For this review, use the dimensioned drawing (mm, ordinates from the lowest corner) and the shaded views. A direction names the side the tool comes from. Coordinates: 2 decimals unless noted, no trailing zeros. Loops run counter-clockwise (first coordinate to the right, second up) from the corner with the lowest first, then second, coordinate; pieces in that order, holes last. Notation, with made-up numbers: M 7,30.5 L 39,30.5 A30 ccw 39,66.5 Z; hole C 76.5,32.25 d8. An arc over 180 degrees is marked long. One line per item, written item: value.
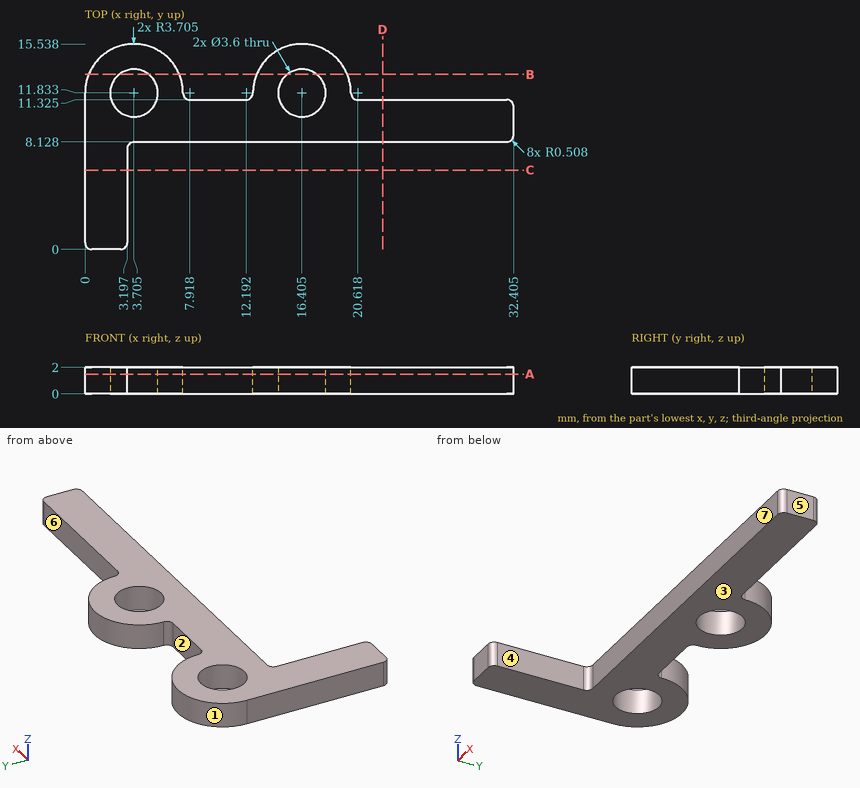
(1) Add section C-C on y = 6. State the section outline as (x, z) points, then the cut area to 3 significant figures.
Checks:
outline: M 0,0 L 3.2,0 L 3.2,2 L 0,2 Z
area: 6.39 mm^2
(2) Add section A-A on z = 1.5. State the section outline as (x, y) points (3 decimals), then the cut area to 3 significant figures.
Checks:
outline: M 0,0.508 A0.508 ccw 0.508,0 L 2.689,0 A0.508 ccw 3.197,0.508 L 3.197,7.62 A0.508 cw 3.705,8.128 L 31.897,8.128 A0.508 ccw 32.405,8.636 L 32.405,10.817 A0.508 ccw 31.897,11.325 L 20.618,11.325 A0.508 cw 20.11,11.833 A3.705 ccw 12.7,11.833 A0.508 cw 12.192,11.325 L 7.918,11.325 A0.508 cw 7.41,11.833 A3.705 ccw 0,11.833 Z; hole C 3.705,11.833 d3.6; hole C 16.405,11.833 d3.6
area: 160 mm^2
(3) Add section D-D on x = 22.5. State the section outline as (y, z) points (3 decimals), then the cut area to 3 significant figures.
Checks:
outline: M 8.128,0 L 11.325,0 L 11.325,2 L 8.128,2 Z
area: 6.39 mm^2
(4) Draft analysis for pull direction X (two halves, no side actions). For the marked faces 1, 2, 3 and 4, state which applies: pulls with the +X half, pulls with the -X half, needs draft (parallel to the pull), parting line crosses it, or undercut.
Checks:
face 1: undercut
face 2: undercut
face 3: needs draft
face 4: pulls with the +X half
(5) Insertion check: pin 1 Ø1 at (x, z) = (11, 1) entering from +Y (3 decimals); pin 2 Ø0.6 at (y, z) = (5.5, 1) entering from +X; pin 3 Ø4 at (x, y) = (12.5, 6) entering from -Z. Each pin has a flat end and moves straight along its axis. Give the tip position at first contact, or say it passes through.
Checks:
pin 1: y = 11.325
pin 2: x = 3.2
pin 3: through
(6) To check wall thickness, follow L1, parallel to X at y = 13, z = 1; L2, parallel to X at y = 10.75, z = 0.45 (3 decimals); L3, parallel to Y at x = 21, z = 0.75 (3 decimals). State the ranges of each line that lie inside material, in increasing order. Write a range as [from, to].
Checks:
L1: [0.19, 2.33], [5.08, 7.22], [12.89, 15.03], [17.78, 19.92]
L2: [0, 2.267], [5.143, 14.967], [17.843, 32.405]
L3: [8.128, 11.325]
(7) Tool access review of the marked faces 5, 6 and 7: name each direction out of +Z, -Z, +X, -X, +Y, -Y from which nothing blocks a thin tool from reaching the whole face with its end or side.
Checks:
face 5: +Z, -Z, +X, +Y, -Y
face 6: +Z, -Z, +X, +Y
face 7: +Z, -Z, +X, -Y
(8) Add section B-B on y = 13.25. State the section outline as (x, z) points (3 decimals).
Checks:
outline: M 0.282,0 L 2.595,0 L 2.595,2 L 0.282,2 Z; M 4.815,0 L 7.128,0 L 7.128,2 L 4.815,2 Z; M 12.982,0 L 15.295,0 L 15.295,2 L 12.982,2 Z; M 17.515,0 L 19.828,0 L 19.828,2 L 17.515,2 Z
